Here's the drawing with two shaded views (mm, measured from the low corner). I have some questions. Give positions to 0.01 mm unless a question says otherwise; leave off trailing zeros. Write each loop counter-clockwise with the first axis right and the second up, starting at its lowest first coordinate (ties: lowest second). Pieces come first, ordered by that corner, then holes. Notation, with made-up numbers: (76, 60.5) - (133, 60.5) arc R31 ccw to (133, 93.5) - close; hole circle Ø11 at (0.5, 84). An arc over 180 degrees is marked (long way). Use one line per item in the form item = value.
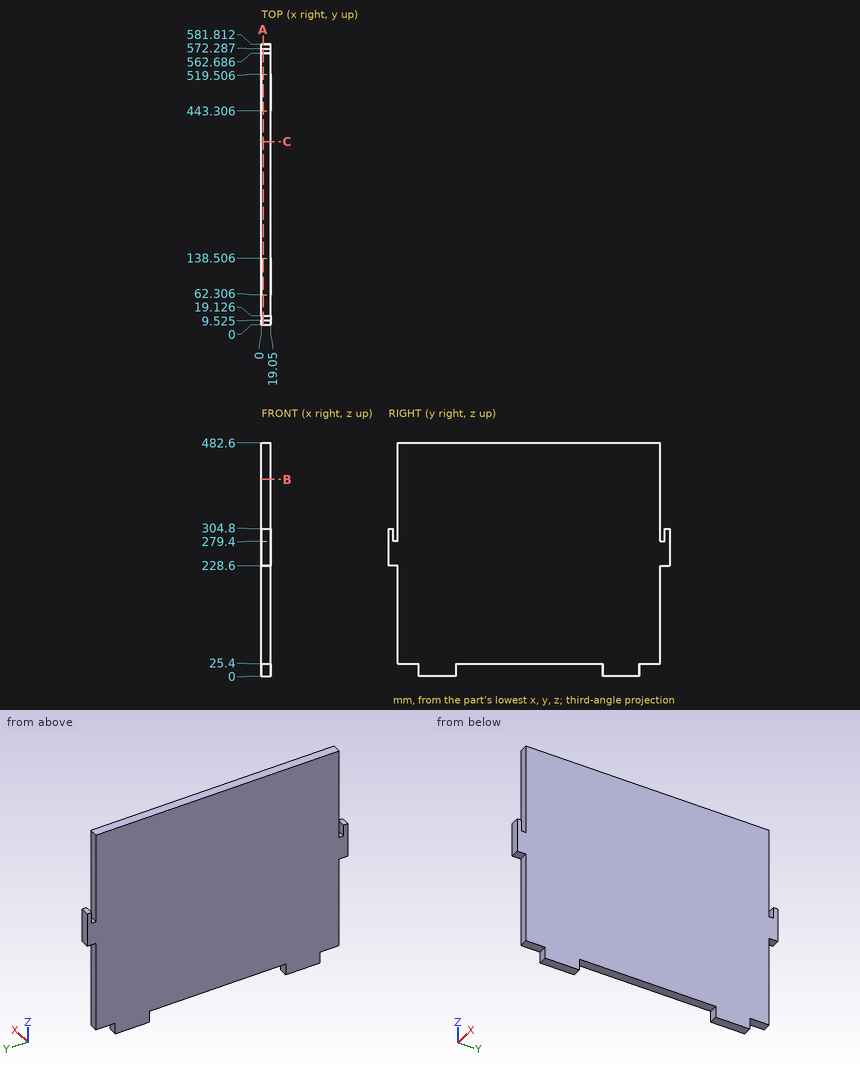
1. For pin 1 (5.5 mm diameter, centred on x = 14, z = 7.5, fed in from +Y); pin 2 (5 mm diameter, centred on x = 6.5, y = 369.5, fed in from -Z); pin 3 (5.5 mm diameter, centred on x = 7, z = 133.5, fed in from +Y); pin 4 (5 mm diameter, centred on y = 329.5, z = 62, fed in from -X), each with a flat end and sliding along its axis, tell me the tip position at first contact or that it passes through.
Response values:
pin_1 = 519.51
pin_2 = 25.4
pin_3 = 562.69
pin_4 = 0
2. Imagine slicing it at C-C, the plane y = 379.5. List the corners of the cut face in (x, z) for me.
Response values:
outline = (0, 25.4) - (19.05, 25.4) - (19.05, 482.6) - (0, 482.6) - close
3. If I drill on line 1 (Y direction, x = 3.25, z = 436); line 2 (Z direction, x = 8, y = 160.5), over which ranges is the centre line in solid material (lowest first)? Write a range as from..to.
Response values:
line_1 = 19.13..562.69
line_2 = 25.4..482.6
4. Imagine slicing it at B-B, the plane z = 407. List the corners of the cut face in (x, y) for me, and give its area (3 significant figures).
Response values:
outline = (0, 19.13) - (19.05, 19.13) - (19.05, 562.69) - (0, 562.69) - close
area = 10,400 mm²
5. Imagine slicing it at A-A, the plane x = 3.5. List the corners of the cut face in (y, z) for me (1 decimal).
Response values:
outline = (0, 228.6) - (19.1, 228.6) - (19.1, 25.4) - (62.3, 25.4) - (62.3, 0) - (138.5, 0) - (138.5, 25.4) - (443.3, 25.4) - (443.3, 0) - (519.5, 0) - (519.5, 25.4) - (562.7, 25.4) - (562.7, 228.6) - (581.8, 228.6) - (581.8, 304.8) - (572.3, 304.8) - (572.3, 279.4) - (562.7, 279.4) - (562.7, 482.6) - (19.1, 482.6) - (19.1, 279.4) - (9.5, 279.4) - (9.5, 304.8) - (0, 304.8) - close
